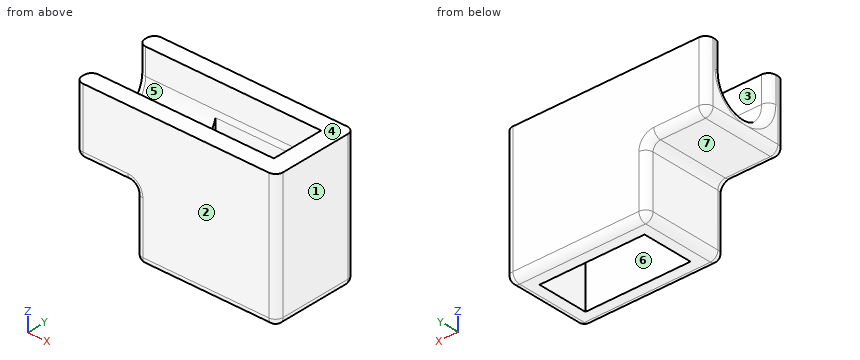
from build123d import *

# Parameters (mm, degrees)
F0_W     = 4
F0_H     = 5.8
F0_W_2   = 9.4
F0_W_3   = 7
F0_H_2   = 3.4
F1_DEPTH = 9
F2_DEPTH = 4.5
F4_DEPTH = 12.2
F5_R     = 0.49999


# Not quite as in the source:
# - a fillet or chamfer is up to 0.001 mm smaller than in the source, because OpenCascade refuses the exact size


with BuildPart() as f1:
    # F0 (on Top) → F1 (new body)
    with BuildSketch(Plane.XY):
        with Locations((-6.7, 0)):
            Rectangle(F0_W, F0_H)
        Rectangle(F0_W_2, F0_H)
        Rectangle(F0_W_3, F0_H_2, mode=Mode.SUBTRACT)
    extrude(amount=F1_DEPTH)

    # F0 (on Top) → F2 (cut)
    with BuildSketch(Plane.XY):
        with Locations((-6.7, 0)):
            Rectangle(F0_W, F0_H)
    extrude(amount=F2_DEPTH, mode=Mode.SUBTRACT)

    # F3 (on face) → F4 (cut, through all)
    with BuildSketch(Plane(origin=(-8.7, 0, 0), x_dir=(0, -1, 0), z_dir=(-1, 0, 0))):
        with BuildLine():
            Line((-1.75, 9), (-1.75, 7.25))
            ThreePointArc((-1.75, 7.25), (0, 5.5), (1.75, 7.25))
            Line((1.75, 7.25), (1.75, 9))
            Line((1.75, 9), (-1.75, 9))
        make_face()
    extrude(amount=-F4_DEPTH, mode=Mode.SUBTRACT)

    # F5 (radius 0.5 in the source; OpenCascade refuses exactly that, so slightly less here)
    f5_edges = [f1.edges().sort_by_distance(p)[0] for p in [
        (-4.7, 2.9, 2.25),
        (-6.7, 2.9, 4.5),
        (-4.7, 0, 4.5),
        (-4.7, -2.9, 2.25),
        (4.7, -2.9, 4.5),
        (4.7, 2.9, 4.5),
        (0, 2.9, 0),
        (4.7, 0, 0),
        (0, -2.9, 0),
        (-4.7, 0, 0),
        (-8.7, 2.9, 6.75),
        (-8.7, 0, 4.5),
        (-8.7, -2.9, 6.75),
        (-8.7, 0, 5.5),
        (-8.7, -1.75, 8.125),
        (-8.7, 1.75, 8.125),
        (-6.7, -2.9, 4.5),
    ]]
    fillet(f5_edges, radius=F5_R)


solid = f1.part
Verification items for the finished model (mm, model axes). Face numbers are marked on the shaded views. A direction names the side the tool comes from. Give positions to 0.01 mm unless a question says otherwise; leave off trailing zeros. Write each loop counter-clockwise with the first axis right and the second up, starting at its lowest first coordinate (ties: lowest second). Pieces come first, ordered by that corner, then holes.
(1) Cross-section at B-B (x = -3). Enter the section's corners in (y, z), plus the area to 3 significant figures.
(2) Cross-section at C-C (z = 1.25). Enter the section's corners in (x, y).
(3) Access from +Z, -Z, +X, -X, +Y, -Y to the whole of each face (thin tool, end or side, straight path). Record for the marked faces 4, 5, 6 and 7.
(4) Gauge pin test, flat ends, axial feed: pin 1 (1.8 mm diameter, centred on y = -1, z = 2.5, fed in from -X); pin 2 (2.5 mm diameter, centred on x = -7, y = 1, fed in from -Z). Record the tip position at first contact, or that the pin passes through.
(5) Mould release check, pull along Y, two halves, no side actions. Record for the marked faces 1, 2 and 3: +Y half, -Y half, draft (parallel to the pull), parting line (faces both ways), or undercut.
(6) Material ranges on line 1 (Y direction, x = 0.5, z = 8.25); line 2 (X direction, y = 1.4, z = 2.75); line 3 (X direction, y = -0.15, z = 6.25), recorded low to high.
Worked out:
1. outline: (-2.9, 0.5) arc R0.5 ccw to (-2.4, 0) - (-1.7, 0) - (-1.7, 6.83) arc R1.75 cw to (-1.75, 7.25) - (-1.75, 9) - (-2.9, 9) - close; (1.7, 0) - (2.4, 0) arc R0.5 ccw to (2.9, 0.5) - (2.9, 9) - (1.75, 9) - (1.75, 7.25) arc R1.75 cw to (1.7, 6.83) - close
1. area: 21.3 mm2
2. outline: (-4.7, -2.4) arc R0.5 ccw to (-4.2, -2.9) - (4.2, -2.9) arc R0.5 ccw to (4.7, -2.4) - (4.7, 2.4) arc R0.5 ccw to (4.2, 2.9) - (-4.2, 2.9) arc R0.5 ccw to (-4.7, 2.4) - close; hole (-3.5, -1.7) - (3.5, -1.7) - (3.5, 1.7) - (-3.5, 1.7) - close
3. face 4: +Z, +X, -X, +Y, -Y
3. face 5: +Z, -X
3. face 6: +Z, -Z
3. face 7: -Z, -X, +Y, -Y
4. pin 1: stops at x = -4.7
4. pin 2: stops at z = 4.5
5. face 1: draft
5. face 2: -Y half
5. face 3: undercut
6. line 1: y = -2.9 to -1.75, 1.75 to 2.9
6. line 2: x = -4.7 to -3.5, 3.5 to 4.7
6. line 3: x = 3.5 to 4.7
